Source: CAD feature listing. Evaluate the final solid. Frame: model axes, mm. A direction names the side the tool comes from. Give positions to 0.01 mm unless a question says otherwise; leave off trailing zeros. Loops run counter-clockwise (first coordinate to the right, second up) from the corner with the lowest first, then second, coordinate; pieces in that order, holes last. Notation, with made-up numbers: (52, 6) -> (89, 6) arc R23 ccw to (89, 26) -> close; hole circle Ø5 at (38, 66). An arc over 180 degrees is marked (long way). Return JSON: item names as keys, results as strings. Group by question number.
(1) Cut plane A-A on z = 12. Return loops of the section in (x, y), then the cut area to 3 significant figures.
(2) Access query for faces 1 (the face through (-10.22, 2.03, 14.4)), 2 (the face through (-11, 4, 20)), 3 (the face through (-4.97, 14.22, 36.9)), 4 (the face through (-3, 10, 20)), 5 (the face through (-9, 0, 20)). Directions: +Z, -Z, +X, -X, +Y, -Y. A direction counts if a zero-diameter tool reaches every point of the face in a straight line with its end or side. Return the directions, or none.
(3) Cut plane C-C on z = 22.5. Return loops of the section in (x, y).
(4) Draft query along Y for faces 6 (the face through (-4.972, 15.807, 36.875)), 7 (the face through (-15, 2, 20)), 8 (the face through (-5, 20, 20)). Return one class per face: released by +Y, released by -Y, zero draft, split by the parting line, or undercut.
(5) Cut plane B-B on x = -3.75. Return loops of the section in (y, z).
(6) Pin query (flat end, axial travel): pin 1 (2 mm diameter, centred on y = 14.5, z = 32, fed in from -X); pin 2 (6.5 mm diameter, centred on x = -11, z = 28, fed in from +Y). Return the tip coordinate at first contact, or that it passes through.
(7) Ray query, line 1 (Y direction, x = -4.1, z = 5.5); line 2 (X direction, y = 1.25, z = 12); line 3 (X direction, y = 15.25, z = 21). Return the intervals inside material, ascending. Write a range as from..to.
(8) Cut plane D-D on y = 6.5. Return loops of the section in (x, z), then the cut area to 3 significant figures.
```python
from build123d import *

# Parameters (mm, degrees)
BOSS_EXTRUDE1_DEPTH = 40
CUT_EXTRUDE1_DEPTH  = 46.617978912
CUT_EXTRUDE2_DEPTH  = 50.839743178
SKETCH8_W           = 6
SKETCH8_H           = 40
CUT_EXTRUDE4_DEPTH  = 46.617978912


with BuildPart() as part:
    # Sketch1 → Boss-Extrude1 (new body)
    with BuildSketch(Plane.XY):
        Polygon((-15, 0), (15, 0), (15, 4), (7, 4), (7, 20), (3, 20), (3, 4), (-3, 4), (-3, 20), (-7, 20), (-7, 4), (-15, 4), align=None)
    extrude(amount=BOSS_EXTRUDE1_DEPTH)

    # Sketch2 → Cut-Extrude1 (cut, through all)
    with BuildSketch(Plane(origin=(0, 4, 0), x_dir=(1, 0, 0), z_dir=(0, 1, 0))):
        with BuildLine():
            Line((-12.590990258, -13.590990258), (-11, -15.181980515))
            Line((-11, -15.181980515), (-9.409009742, -13.590990258))
            ThreePointArc((-9.409009742, -13.590990258), (-11, -9.75), (-12.590990258, -13.590990258))
        make_face()
        with BuildLine():
            Line((9.409009742, -13.590990258), (11, -15.181980515))
            Line((11, -15.181980515), (12.590990258, -13.590990258))
            ThreePointArc((12.590990258, -13.590990258), (11, -9.75), (9.409009742, -13.590990258))
        make_face()
    extrude(amount=-CUT_EXTRUDE1_DEPTH, mode=Mode.SUBTRACT)

    # Sketch3 → Cut-Extrude2 (cut, through all)
    with BuildSketch(Plane(origin=(7, 0, 0), x_dir=(0, 0, -1), z_dir=(1, 0, 0))):
        with BuildLine():
            Line((-7.090990258, 16.590990258), (-8.681980515, 15))
            Line((-8.681980515, 15), (-7.090990258, 13.409009742))
            ThreePointArc((-7.090990258, 13.409009742), (-3.25, 15), (-7.090990258, 16.590990258))
        make_face()
        with BuildLine():
            Line((-36.090990258, 16.590990258), (-37.681980515, 15))
            Line((-37.681980515, 15), (-36.090990258, 13.409009742))
            ThreePointArc((-36.090990258, 13.409009742), (-32.25, 15), (-36.090990258, 16.590990258))
        make_face()
    extrude(amount=-CUT_EXTRUDE2_DEPTH, mode=Mode.SUBTRACT)

    # Sketch8 → Cut-Extrude4 (cut, through all)
    with BuildSketch(Plane(origin=(0, 4, 0), x_dir=(1, 0, 0), z_dir=(0, 1, 0))):
        with Locations((0, -20)):
            Rectangle(SKETCH8_W, SKETCH8_H)
    extrude(amount=-CUT_EXTRUDE4_DEPTH, mode=Mode.SUBTRACT)


with BuildPart() as cut_extrude4_piece_1:
    # of the separate pieces the step leaves, piece 1, a body of its own (cut_extrude4_pieces)
    add(part.part.solids().sort_by_distance((-15, 0, 0))[0])


with BuildPart() as cut_extrude4_piece_2:
    # of the separate pieces the step leaves, piece 2, a body of its own (cut_extrude4_pieces)
    add(part.part.solids().sort_by_distance((3, 0, 0))[0])


solid = cut_extrude4_piece_1.part
```
Answers:
{
 "1": {"outline": "(-15, 0) -> (-13.25, 0) -> (-13.25, 4) -> (-15, 4) -> close; (-8.75, 0) -> (-3, 0) -> (-3, 20) -> (-7, 20) -> (-7, 4) -> (-8.75, 4) -> close", "area": "94.0 mm²"},
 "2": {"face 1": "+Y, -Y", "face 2": "+Z, -Z, -X, +Y", "face 3": "+X, -X", "face 4": "+Z, -Z, +X, +Y, -Y", "face 5": "+Z, -Z, +X, -X, -Y"},
 "3": {"outline": "(-15, 0) -> (-3, 0) -> (-3, 20) -> (-7, 20) -> (-7, 4) -> (-15, 4) -> close"},
 "4": {"face 6": "undercut", "face 7": "zero draft", "face 8": "released by +Y"},
 "5": {"outline": "(0, 0) -> (20, 0) -> (20, 40) -> (0, 40) -> close; hole (13.41, 7.09) arc R2.25 ccw (long way) to (16.59, 7.09) -> (15, 8.68) -> close; hole (13.41, 36.09) arc R2.25 ccw (long way) to (16.59, 36.09) -> (15, 37.68) -> close"},
 "6": {"pin 1": "x = -7", "pin 2": "y = 4"},
 "7": {"line 1": "0..12.75, 17.25..20", "line 2": "-15..-13.25, -8.75..-3", "line 3": "-7..-3"},
 "8": {"outline": "(-7, 0) -> (-3, 0) -> (-3, 40) -> (-7, 40) -> close", "area": "160 mm²"}
}
